Autodesk Inventor part; units mm, degrees
ref_plane "Plano de trabajo1" through (106, -5, -152) normal (0, 0, -1) x (-1, 0, 0)
ref_plane "Plano de trabajo2" through (-50, -5, -157) normal (1, 0, 0) x (0, 0, -1)
ref_plane "YZ Plane" through (0, 0, 0) normal (1, 0, 0) x (0, 1, 0)
sketch "Boceto1" plane through (0, 0, 0) normal (0, 0, 1) x (1, 0, 0)
  line L0 (0, 0) -> (100, 0)
  line L1 (0, 300.0017) -> (0, 100.0017)
  line L2 (0, 0) -> (101, 0)
  line L3 (101, 0) -> (101, 400)
  line L4 (101, 400) -> (0, 400)
  line L5 (0, 300.0017) -> (0, 100.0017)
  line L6 (0, 0) -> (98.1777, 0) construction
  line L7 (98.1777, 0) -> (98.1777, 330) construction
  line L8 (98.1777, 330) -> (0, 330) construction
  line L9 (0, 330) -> (0, 0) construction
  line L10 (0, 300.0017) -> (-100, 300.0017) construction
  line L11 (-100, 300.0017) -> (-100, 100.0017) construction
  line L12 (-100, 100.0017) -> (0, 100.0017) construction
  line L13 (0, 100.0017) -> (0, 300.0017) construction
  line L14 (0, 300.0017) -> (-100, 300.0017)
  line L15 (-100, 300.0017) -> (-100, 100.0017)
  line L16 (-100, 100.0017) -> (0, 100.0017)
  line L17 (0, 100.0017) -> (0, 300.0017)
  line L18 (-100, 0) -> (-201, 0)
  line L19 (-201, 0) -> (-201, 400)
  line L20 (-201, 400) -> (-100, 400)
  line L21 (-100, 300.0017) -> (-100, 100.0017)
  line L22 (-100, 0) -> (0, 0)
  line L23 (-100, 400) -> (0, 400)
  line L24 (-95, 105.0017) -> (-5, 105.0017)
  line L25 (-5, 105.0017) -> (-5, 295.0017)
  line L26 (-5, 295.0017) -> (-95, 295.0017)
  line L27 (-95, 295.0017) -> (-95, 105.0017)
  line L28 (106, 400) -> (106, -5)
  line L29 (106, -5) -> (-206, -5)
  line L30 (-206, -5) -> (-206, 400)
  line L31 (-206, 400) -> (-201, 400)
  line L32 (101, 400) -> (106, 400)
  line L33 (-100, 100.0017) -> (-100, 0) construction
  line L34 (-50, -5) -> (-50, -60) construction
  arc A0 (-61.35, -74.5956) -> (-206, -5) centre (-205.942, -190) ccw
  arc A1 (106, -5) -> (-38.65, -74.5956) centre (105.942, -190) ccw
  line L35 (-38.65, -74.5956) -> (-38.65, -69.5956)
  line L36 (-61.35, -74.5956) -> (-61.35, -69.5956)
  line L37 (-61.35, -69.5956) -> (-38.65, -69.5956)
  line L38 (-100, 0) -> (-100, -33.3083)
  line L39 (0, 0) -> (0, -33.2635)
  line L40 (-100, 400) -> (-100, 300.0017) construction
  line L41 (-69.5521, -60) -> (-30.4598, -60)
  line L42 (-50, -65) -> (-30.4399, -65)
  line L43 (-30.4399, -65) -> (-69.5601, -65)
  arc A2 (98.1777, 0) -> (-30.4598, -60) centre (106.0764, -184.8313) ccw
  arc A3 (-69.5521, -60) -> (-201, 0) centre (-205.9958, -184.9325) ccw
  point P0 (-162.9925, -5)
  point P1 (-100, -5)
  point P2 (62.6517, -5)
  point P3 (0, -5)
  dimension "d2" = 101
  dimension "d9" = 101
  dimension "d11" = 400
  dimension "d12" = 100
  dimension "d13" = 200
  dimension "d14" = 100
  dimension "d15" = 5
  dimension "d16" = 5
  dimension "d17" = 5
  dimension "d18" = 5
  dimension "d19" = 5
  dimension "d20" = 5
  dimension "d22" = 55
  dimension "d27" = 302
  dimension "d30" = 185
  dimension "d31" = 185
  dimension "d33" = 5
  dimension "d36" = 5
  dimension "d120" = 5
extrude "Extrusión1" add sketch "Boceto1" against normal blind 152 contours L30 L31 L19 A3 L29 | L0 L2 L3 L32 L28 L29 A2 | L38 L29 A3 L18 | L29 A2 L39 | L29 A1 L42 L43 A0 A3 L41 A2 | L38 A3 L29 | A1 L35 L37 L36 A0 L43 L42 | L1 L16 L15 L14
sketch "Boceto2" plane through (0, 0, 0) normal (0, 0, 1) x (1, 0, 0)
  line L0 (-206, 400) -> (-206, -5)
  line L1 (106, -5) -> (106, 400)
  arc A0 (106, -5) -> (-38.65, -74.5956) centre (105.942, -190) ccw
  arc A1 (-61.35, -74.5956) -> (-206, -5) centre (-205.942, -190) ccw
  line L2 (-61.35, -74.5956) -> (-38.65, -74.5956)
  line L3 (-206, 400) -> (106, 400)
  line L4 (-201, 0) -> (-201, 400)
  line L5 (0, 300.0017) -> (-100, 300.0017)
  line L6 (0, 100.0017) -> (0, 300.0017)
  line L7 (-95, 105.0017) -> (-95, 295.0017)
  line L8 (-5, 295.0017) -> (-5, 105.0017)
  line L9 (-5, 105.0017) -> (-95, 105.0017)
  line L10 (-95, 295.0017) -> (-5, 295.0017)
  point P0 (0, 0)
extrude "Extrusión2" add sketch "Boceto2" along normal blind 5
ref_plane "Plano de trabajo1" through (106, -5, -152) normal (0, 0, -1) x (-1, 0, 0)
sketch "Boceto5" plane through (106, -5, -152) normal (0, 0, -1) x (-1, 0, 0)
  line L0 (312, 0) -> (312, 405)
  line L1 (312, 405) -> (307, 405)
  line L2 (5, 405) -> (307, 405)
  line L3 (5, 405) -> (0, 405)
  line L4 (0, 405) -> (0, 0)
  arc A0 (144.65, -69.5956) -> (0, 0) centre (0.058, -185) ccw
  line L5 (144.65, -69.5956) -> (167.35, -69.5956)
  arc A1 (312, 0) -> (167.35, -69.5956) centre (311.942, -185) ccw
  line L6 (201, 110.0017) -> (111, 110.0017)
  line L7 (111, 110.0017) -> (111, 300.0017)
  line L8 (111, 300.0017) -> (201, 300.0017)
  line L9 (201, 300.0017) -> (201, 110.0017)
  point P0 (106, 5)
extrude "Extrusión3" add sketch "Boceto5" along normal blind 5
sketch "Boceto7" plane through (-206, -5, 5) normal (-1, 0, 0) x (0, 0, 1)
  line L0 (-162, 0) -> (0, 0) construction
  line L1 (-81, 0) -> (-81, 5) construction
  line L2 (-81, 5) -> (-81, 35) construction
  line L3 (-81, 35) -> (-81, 115) construction
  line L4 (-81, 115) -> (-81, 145) construction
  line L5 (-81, 145) -> (-81, 225) construction
  line L6 (-81, 225) -> (-81, 255) construction
  line L7 (-81, 255) -> (-81, 335) construction
  line L8 (-157, 35) -> (-5, 35)
  line L9 (-5, 35) -> (-5, 115)
  line L10 (-5, 115) -> (-157, 115)
  line L11 (-157, 115) -> (-157, 35)
  line L12 (0, 405) -> (0, 0)
  line L13 (-162, 0) -> (-162, 405)
  line L14 (-5, 225) -> (-157, 225)
  line L15 (-157, 225) -> (-157, 145)
  line L16 (-157, 145) -> (-5, 145)
  line L17 (-5, 145) -> (-5, 225)
  line L18 (-5, 335) -> (-157, 335)
  line L19 (-157, 335) -> (-157, 255)
  line L20 (-157, 255) -> (-5, 255)
  line L21 (-5, 255) -> (-5, 335)
  point P0 (-5, 5)
  dimension "d47" = 5
  dimension "d48" = 30
  dimension "d49" = 80
  dimension "d50" = 30
  dimension "d51" = 80
  dimension "d52" = 30
  dimension "d53" = 80
  dimension "d54" = 5
  dimension "d55" = 5
  dimension "d58" = 110
sketch "Boceto8" plane through (106, -5, 5) normal (1, 0, 0) x (0, 0, -1)
  line L0 (5, 335) -> (157, 335)
  line L1 (157, 335) -> (157, 255)
  line L2 (157, 255) -> (5, 255)
  line L3 (5, 255) -> (5, 335)
  line L4 (5, 225) -> (157, 225)
  line L5 (157, 225) -> (157, 145)
  line L6 (157, 145) -> (5, 145)
  line L7 (5, 145) -> (5, 225)
  line L8 (5, 115) -> (157, 115)
  line L9 (157, 115) -> (157, 35)
  line L10 (157, 35) -> (5, 35)
  line L11 (5, 35) -> (5, 115)
  point P0 (5, 5)
extrude "Extrusión5" cut sketch "Boceto7" against normal blind 5
extrude "Extrusión6" cut sketch "Boceto8" against normal blind 5
sketch "Boceto9" plane through (106, -5, -152) normal (0, 0, 1) x (1, 0, 0)
  line L0 (0, 405) -> (0, 0) construction
  line L1 (0, 372.4568) -> (-312, 372.4568) construction
  line L2 (-312, 0) -> (-312, 405) construction
  line L3 (-156, 372.4568) -> (-156, 300.0017) construction
  line L4 (-111, 300.0017) -> (-201, 300.0017) construction
  line L5 (-312, 405) -> (0, 405) construction
  line L6 (-156, 405) -> (-156, 385) construction
  line L7 (-106, 405) -> (-106, 305) construction
  line L8 (-106, 305) -> (-206, 305) construction
  line L9 (-206, 305) -> (-106, 305)
  line L10 (-206, 305) -> (-156, 367.45)
  line L11 (-106, 305) -> (-156, 367.45)
  point P0 (-106, 5)
  dimension "d71" = 20
  dimension "d72" = 100
  dimension "d73" = 80
extrude "Extrusión7" add sketch "Boceto9" along normal blind 152
sketch "Boceto11" plane through (106, -5, 5) normal (1, 0, 0) x (0, 0, -1)
  line L0 (157, 405) -> (157, 335)
  line L1 (5, 350) -> (157, 350)
  line L2 (157, 350) -> (157, 365)
  line L3 (157, 365) -> (5, 365)
  line L4 (5, 365) -> (5, 350)
  line L5 (5, 105.0017) -> (5, 305.0017)
  line L6 (5, 10) -> (157, 10)
  line L7 (157, 10) -> (157, 25)
  line L8 (157, 25) -> (5, 25)
  line L9 (5, 25) -> (5, 10)
  line L10 (162, 405) -> (0, 405)
  line L11 (157, 35) -> (5, 35)
  line L12 (0, 405) -> (0, 0)
  line L13 (5, 122.5) -> (0, 122.5)
  line L14 (0, 122.5) -> (0, 137.5)
  line L15 (0, 137.5) -> (5, 137.5)
  line L16 (5, 137.5) -> (5, 122.5)
  line L17 (5, 232.5) -> (0, 232.5)
  line L18 (0, 232.5) -> (0, 247.5)
  line L19 (0, 247.5) -> (5, 247.5)
  line L20 (5, 247.5) -> (5, 232.5)
  line L21 (157, 255) -> (5, 255)
  line L22 (5, 225) -> (157, 225)
  line L23 (157, 145) -> (5, 145)
  line L24 (5, 115) -> (157, 115)
  point P0 (5, 5)
  dimension "d79" = 152
  dimension "d80" = 40
  dimension "d81" = 15
  dimension "d84" = 15
  dimension "d89" = 10
  dimension "d92" = 7.5
  dimension "d93" = 7.5
  dimension "d94" = 7.5
  dimension "d95" = 7.5
extrude "Extrusión8" add sketch "Boceto11" along normal blind 3 contours L0 L1 L4 L3 | L19 L5 L17 L12 | L15 L5 L13 L12 | L9 L8 L7 L6
sketch "Boceto12" plane through (106, 345, -152) normal (0, -1, 0) x (1, 0, 0)
  line L0 (1, 152) -> (2, 152)
  line L1 (2, 152) -> (2, 0)
  line L2 (2, 0) -> (1, 0)
  line L3 (1, 0) -> (1, 152)
  line L4 (0, 152) -> (0, 0)
  line L5 (0, 152) -> (3, 152)
  line L6 (0, 0) -> (3, 0)
  point P0 (-106, 152)
  dimension "d96" = 1
  dimension "d97" = 1
  dimension "d98" = 0
  dimension "d99" = 0
extrude "Extrusión9" cut sketch "Boceto12" against normal blind 5 contours L0 L1 L2 L3
sketch "Boceto13" plane through (106, 20, 0) normal (0, 1, 0) x (1, 0, 0)
  line L0 (2, 0) -> (1, 0)
  line L1 (1, 0) -> (1, 152)
  line L2 (1, 152) -> (2, 152)
  line L3 (2, 152) -> (2, 0)
  line L4 (0, 0) -> (3, 0)
  line L5 (0, 0) -> (0, 152)
  line L6 (0, 152) -> (3, 152)
  point P0 (-106, 0)
  dimension "d102" = 0
  dimension "d103" = 1
  dimension "d104" = 1
  dimension "d105" = 0
extrude "Extrusión10" cut sketch "Boceto13" against normal blind 5 contours L0 L1 L2 L3
ref_plane "Plano de trabajo2" through (-50, -5, -157) normal (1, 0, 0) x (0, 0, -1)
mirror "Simetría1" about plane through (-50, -5, -157) normal (1, 0, 0) of "Extrusión8"
sketch "Boceto14" plane through (-206, 20, 0) normal (0, 1, 0) x (1, 0, 0)
  line L0 (-2, 152) -> (-1, 152)
  line L1 (-1, 152) -> (-1, 0)
  line L2 (-1, 0) -> (-2, 0)
  line L3 (-2, 0) -> (-2, 152)
  line L4 (0, 152) -> (-3, 152)
  line L5 (-3, 152) -> (-3, 0)
  line L6 (0, 0) -> (-3, 0)
  point P0 (206, 0)
  dimension "d108" = 0
  dimension "d109" = 1
  dimension "d110" = 1
  dimension "d111" = 0
extrude "Extrusión11" cut sketch "Boceto14" against normal blind 5 contours L0 L1 L2 L3
sketch "Boceto15" plane through (-206, 345, -152) normal (0, -1, 0) x (1, 0, 0)
  line L0 (-1, 0) -> (-2, 0)
  line L1 (-2, 0) -> (-2, 152)
  line L2 (-2, 152) -> (-1, 152)
  line L3 (-1, 152) -> (-1, 0)
  line L4 (0, 0) -> (-3, 0)
  line L5 (-3, 0) -> (-3, 152)
  line L6 (0, 152) -> (-3, 152)
  point P0 (206, 152)
  dimension "d114" = 0
  dimension "d115" = 1
  dimension "d116" = 1
  dimension "d117" = 0
extrude "Extrusión12" cut sketch "Boceto15" against normal blind 5 contours L0 L1 L2 L3
sketch "Sketch16" plane through (-61.35, -69.5956, 0) normal (0, -1, 0) x (1, 0, 0)
  line L0 (11.35, -152) -> (11.35, 0)
  circle A0 centre (11.35, -76) radius 15
  point P0 (61.35, 0)
  dimension "d121" = 30
extrude "Extrusion13" cut sketch "Sketch16" along normal mid plane 30
sketch "Sketch17" plane through (106, -5, -157) normal (0, 0, -1) x (-1, 0, 0)
  line L0 (131, -44.5956) -> (120.5222, -44.5956)
  arc A0 (144.65, -69.5956) -> (0, 0) centre (0.058, -185) ccw
  line L1 (181, -44.5956) -> (191.4778, -44.5956)
  arc A1 (312, 0) -> (167.35, -69.5956) centre (311.942, -185) ccw
  line L2 (191.4778, -44.5956) -> (120.5218, -44.5956)
  line L3 (120.5218, -44.5956) -> (120.5218, -69.5956)
  line L4 (120.5218, -69.5956) -> (191.4778, -69.5956)
  line L5 (191.4778, -69.5956) -> (191.4778, -44.5956)
  line L6 (167.35, -69.5956) -> (144.65, -69.5956)
  line L7 (156, -69.5956) -> (120.5218, -69.5956)
  line L8 (167.35, -69.5956) -> (144.65, -69.5956)
  point P0 (106, 5)
  point P1 (155.7098, -69.5956)
  point P2 (144.65, -69.5956)
  point P3 (167.35, -69.5956)
  dimension "d124" = 50
  dimension "d134" = 25
  dimension "d135" = 70.956
  dimension "d136" = 35.4778
  dimension "d137" = 35.188
extrude "Extrusion14" cut sketch "Sketch17" against normal blind 200 contours L2 L1 A1 L4 A0 L0
sketch "Sketch18" plane through (-85.4778, -49.5956, -157) normal (0, -1, 0) x (1, 0, 0)
  point P0 (85.4778, 157)
sketch "Sketch19" plane through (-85.4778, -49.5956, -157) normal (0, -1, 0) x (1, 0, 0)
  line L0 (191.4778, 162) -> (-120.5222, 162)
  line L1 (0, 0) -> (-120.5222, 0)
  line L2 (70.7311, 162) -> (0, 162)
  line L3 (0, 162) -> (0, 0)
  line L4 (0, 0) -> (70.7311, 0)
  line L5 (70.7311, 0) -> (70.7311, 162)
  point P0 (85.4778, 157)
extrude "Extrusion15" add sketch "Sketch19" against normal blind 5
sketch "Sketch20" plane through (-85.4778, -49.5956, -157) normal (0, -1, 0) x (1, 0, 0)
  circle A0 centre (35.4778, 81) radius 25
  line L0 (70.9556, 0) -> (0, 0)
  line L1 (0, 162) -> (70.9556, 162)
  line L2 (191.4778, 162) -> (-120.5222, 162)
  line L3 (35.4778, 162) -> (35.4778, 81)
  line L4 (35.4778, 5) -> (35.4778, 157)
  point P0 (85.4778, 157)
  dimension "d129" = 50
  dimension "d138" = 162
  dimension "d139" = 81
extrude "Extrusion16" cut sketch "Sketch20" against normal blind 10
equation "\"d16\" = d15"
equation "\"d17\" = d15"
equation "\"d18\" = d15"
equation "\"d19\" = d15"
equation "\"d20\" = d15"
equation "\"d31\" = d30"
equation "\"d84\" = d81"
properties part number "Contenedor" material "Acrylic"
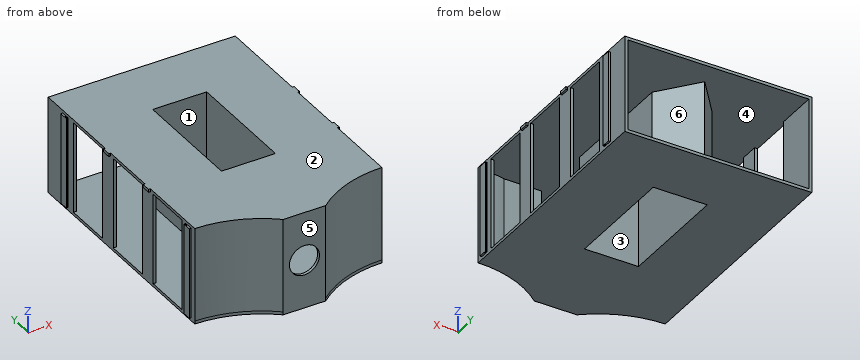
Source: CAD feature listing. Evaluate the final solid. Frame: model axes, mm. Face numbers are marked on the shaded views. A direction names the side the tool comes from. Give positions to 0.01 mm unless a question says otherwise; leave off trailing zeros. Loops run counter-clockwise (first coordinate to the right, second up) from the corner with the lowest first, then second, coordinate; pieces in that order, holes last. Notation, with made-up numbers: (30, 31.5) - (41, 31.5) arc R27 cw to (41, 68.5) - close; hole circle Ø8 at (-20, 26.5). An arc over 180 degrees is marked (long way). Use CSV: the item, a comma, the result in double quotes. Start each with the question number.
1. Ray query, L1, parallel to X at y = 136, z = -7.5; L2, parallel to Z at x = -50, y = -48.2; L3, parallel to Z at x = 59.5, y = 245.5. Return the intervals inside material, ascending.
2. Pin query (flat end, axial travel): pin 1 (6 mm diameter, centred on y = 257, z = -117, fed in from -X); pin 2 (8 mm diameter, centred on x = 34.5, z = -72, fed in from +Y); pin 3 (2 mm diameter, centred on y = 284, z = -14, fed in from +X); pin 4 (3.5 mm diameter, centred on x = 107.5, y = 352, fed in from +Z). Return the tip coordinate at first contact, or that it passes through.
3. Section A-A (y = 154). Output: boundary loops of the cut face in (x, z).
4. Section B-B (y = 371). Output: boundary loops of the cut face in (x, z), then the cut area to 3 significant figures.
5. Section D-D (z = -13). Count the separate pieces of the cut face and the enclosed holes in it, then the cut area to 3 significant figures.
6. Section C-C (x = -41). Output: boundary loops of the cut face in (y, z).
7. Reachability of the marked faces 3, 4, 5 and 6 from +Z, -Z, +X, -X, +Y, -Y: full face, straight path, thin tool, end or side. Return the list, or none.
8. Draft query along X for the marked faces 1 and 2. Return one class per face: +X half, -X half, draft (parallel to the pull), parting line (faces both ways), or undercut.
Response:
1,L1,"-206 to -201, -100 to -95, -5 to 0, 101 to 106"
1,L2,"-157 to -101, -51 to 5"
1,L3,"-157 to -152, 0 to 5"
2,pin 1,"x = -100"
2,pin 2,"y = -5"
2,pin 3,"x = 0"
2,pin 4,"z = 5"
3,outline,"(-206, -157) - (-95, -157) - (-95, 5) - (-206, 5) - (-206, 0) - (-100, 0) - (-100, -152) - (-206, -152) - close; (-5, -157) - (106, -157) - (106, -152) - (0, -152) - (0, 0) - (106, 0) - (106, 5) - (-5, 5) - close"
4,outline,"(-206, -157) - (106, -157) - (106, 5) - (-206, 5) - close; hole (-201, -152) - (101, -152) - (101, 0) - (-201, 0) - close"
4,area,"4,640 mm²"
5,separate pieces,"8"
5,enclosed holes,"1"
5,area,"11,200 mm²"
6,outline,"(-49.6, -157) - (105, -157) - (105, 5) - (-49.6, 5) - (-49.6, -52.68) - (-44.6, -52.68) - (-44.6, 0) - (100, 0) - (100, -152) - (-44.6, -152) - (-44.6, -99.32) - (-49.6, -99.32) - close; (295, -157) - (400, -157) - (400, -152) - (351.21, -152) - (351.21, 0) - (400, 0) - (400, 5) - (295, 5) - close"
7,face 3,"+Z, -Z"
7,face 4,"none"
7,face 5,"+Z, -Z, +X, -X, -Y"
7,face 6,"+Y"
8,face 1,"undercut"
8,face 2,"draft"
